Here's how the part is built. I have some questions about the finished solid (model axes, mm). A direction names the side the tool comes from. Coordinates: 2 decimals unless noted, no trailing zeros. Write each loop counter-clockwise with the first axis right and the second up, starting at its lowest first coordinate (ties: lowest second). Pieces come first, ordered by that corner, then holes. Notation, with made-up numbers: (79, 45) - (99, 45) arc R12 ccw to (99, 67) - close; hole circle Ø6 at (-34, -30.75). An arc over 180 degrees is marked (long way). Answer in a Markdown table with one row per item. Add a question column.
Item 1: I'm going to push flat-ended pins straight in: pin 1 (3 mm diameter, centred on x = 2, z = -57, fed in from +Y); pin 2 (6 mm diameter, centred on x = -2.5, y = 86, fed in from +Z); pin 3 (3 mm diameter, centred on x = 1.5, z = -199, fed in from -Y); pin 4 (3 mm diameter, centred on x = 1.5, y = 30, fed in from -Z). Where does each tip first touch, or does it pass through?
Item 2: Imagine slicing it at B-B (y = 57). Please give me the cut outline in (x, z).
Item 3: We'd pull the mould along Y, two halves only. Please class faces 3 (the face through (0.07, 7.54, -156.01)), 4 (the face through (0.07, 140.003, -241.695)), 5 (the face through (0, 20, -61)), 6 (the face through (-0.07, 81.438, -67.325)): +Y half, -Y half, draft (parallel to the pull), parting line (faces both ways), or undercut.
Item 4: Which directions (+Z, -Z, +X, -X, +Y, -Y) give clear straight access to the entire face, cutting with the end or side of a thin tool? Please do faces 1 (the face through (-0.07, 77.45, -37.26)), 2 (the face through (0.07, 144.455, -121.625)).
Item 5: Imagine slicing it at A-A (z = -275). Please give me the cut outline in (x, y).
Item 6: If I drill on probe 1 along Y at (x, z) = (-2, -70); probe 2 along Z at (x, y) = (0.5, 36); probe 3 along Z at (x, y) = (2.75, 62.5), over which ranges is the centre line in solid material (lowest first)? Write a range as from..to.
Item 7: Imagine slicing it at C-C (x = -1.25). State how many separate pieces and enclosed holes the cut face has, plus the area to 3 significant figures.
from build123d import *

# Parameters (mm, degrees)
ESQUISSE1_W                  = 300
ESQUISSE1_H                  = 150
BOSS_EXTRU_1_DEPTH           = 5
ESQUISSE2_OUTSIDE_W          = 369.112
ESQUISSE2_OUTSIDE_H          = 219.112
ENL_V_MAT_EXTRU_1_DEPTH      = 5
ENL_V_MAT_EXTRU_2_DEPTH      = 336.559234711
ENL_V_MAT_EXTRU_2_DEPTH_BACK = 336.559234711
ENL_V_MAT_EXTRU_3_DEPTH      = 336.559234711
ENL_V_MAT_EXTRU_3_DEPTH_BACK = 336.559234711
ENL_V_MAT_EXTRU_4_DEPTH      = 336.559234711
ENL_V_MAT_EXTRU_4_DEPTH_BACK = 336.559234711
ESQUISSE5_R                  = 10
ESQUISSE6_W                  = 20
ESQUISSE6_H                  = 10
ENL_V_MAT_EXTRU_5_DEPTH      = 49


with BuildPart() as part:
    # Esquisse1 → Boss.-Extru.1 (new, symmetric)
    with BuildSketch(Plane(origin=(0, 0, 0), x_dir=(0, 0, -1), z_dir=(1, 0, 0))):
        with Locations((150, 75)):
            Rectangle(ESQUISSE1_W, ESQUISSE1_H)
    extrude(amount=BOSS_EXTRU_1_DEPTH, both=True)

    # Esquisse2 outside → Enlèv. mat.-Extru.1 (cut, symmetric)
    with BuildSketch(Plane(origin=(0, 0, 0), x_dir=(0, 0, -1), z_dir=(1, 0, 0))):
        with Locations((150, 75)):
            Rectangle(ESQUISSE2_OUTSIDE_W, ESQUISSE2_OUTSIDE_H)
        Polygon((0, 117.225703003), (60, 139.063917059), (185, 150), (300, 129.722397219), (300, 99.722397219), (211.741963761, 84.160124165), (171.741963761, 14.878091862), (139.835792798, 0), (29.835792798, 0), (0, 17.225703003), align=None, mode=Mode.SUBTRACT)
    extrude(amount=ENL_V_MAT_EXTRU_1_DEPTH, both=True, mode=Mode.SUBTRACT)

    # Esquisse3 → Enlèv. mat.-Extru.2 (cut, two sides: drawn at the far end of the back side and taken through both)
    with BuildSketch(Plane(origin=(5, 0, 0), x_dir=(0, 0, -1), z_dir=(1, 0, 0)).offset(-ENL_V_MAT_EXTRU_2_DEPTH_BACK)):
        Polygon((20, 103.221552239), (20, 80.493304508), (55, 74.321860183), (80, 88.755616913), (62.679491924, 118.755616913), align=None)
        Polygon((90, 71.435108837), (113.922571241, 30), (81.508057782, 49.831775443), align=None)
        Polygon((82.886751346, 123.755616913), (139.903333355, 25), (175.32640016, 86.354551467), (150.32640016, 129.655821657), align=None)
        Polygon((91.944969354, 20), (30, 20), (30, 48.267236345), (52.117107943, 44.367393479), align=None)
    extrude(amount=ENL_V_MAT_EXTRU_2_DEPTH + ENL_V_MAT_EXTRU_2_DEPTH_BACK, mode=Mode.SUBTRACT)

    # Esquisse4 → Enlèv. mat.-Extru.3 (cut, two sides: drawn at the far end of the back side and taken through both)
    with BuildSketch(Plane(origin=(5, 0, 0), x_dir=(0, 0, -1), z_dir=(1, 0, 0)).offset(-ENL_V_MAT_EXTRU_3_DEPTH_BACK)):
        Polygon((0, 97.225703003), (3, 97.225703003), (5, 99.225703003), (5, 91.225703003), (3, 93.225703003), (0, 93.225703003), align=None)
        Polygon((3, 41.225703003), (0, 41.225703003), (0, 37.225703003), (3, 37.225703003), (5, 35.225703003), (5, 43.225703003), align=None)
    extrude(amount=ENL_V_MAT_EXTRU_3_DEPTH + ENL_V_MAT_EXTRU_3_DEPTH_BACK, mode=Mode.SUBTRACT)

    # Esquisse5 → Enlèv. mat.-Extru.4 (cut, two sides: drawn at the far end of the back side and taken through both)
    with BuildSketch(Plane.ZY.offset(5).offset(-ENL_V_MAT_EXTRU_4_DEPTH_BACK)):
        with Locations((-275, 114.722397219)):
            Circle(ESQUISSE5_R)
    extrude(amount=ENL_V_MAT_EXTRU_4_DEPTH + ENL_V_MAT_EXTRU_4_DEPTH_BACK, mode=Mode.SUBTRACT)

    # Esquisse6 → Enlèv. mat.-Extru.5 (cut)
    with BuildSketch(Plane(origin=(5, 0, 0), x_dir=(0, 0, -1), z_dir=(1, 0, 0))):
        with Locations((195, 128)):
            Rectangle(ESQUISSE6_W, ESQUISSE6_H)
    extrude(amount=-ENL_V_MAT_EXTRU_5_DEPTH, mode=Mode.SUBTRACT)


solid = part.part
Here are the results:
| question | item | result |
|---|---|---|
| 1 | pin 1 | stops at y = 138.52 |
| 1 | pin 2 | stops at z = 0 |
| 1 | pin 3 | stops at y = 59.49 |
| 1 | pin 4 | stops at z = -181.34 |
| 2 | outline | (-5, -196.06) - (5, -196.06) - (5, -158.38) - (-5, -158.38) - close; (-5, -121.43) - (5, -121.43) - (5, -98.33) - (-5, -98.33) - close; (-5, -84.33) - (5, -84.33) - (5, 0) - (-5, 0) - close |
| 3 | face 3 | -Y half |
| 3 | face 4 | +Y half |
| 3 | face 5 | undercut |
| 3 | face 6 | undercut |
| 4 | face 1 | +X, -X |
| 4 | face 2 | +Z, +X, -X, +Y |
| 5 | outline | (-5, 95.31) - (5, 95.31) - (5, 104.72) - (-5, 104.72) - close; (-5, 124.72) - (5, 124.72) - (5, 134.13) - (-5, 134.13) - close |
| 6 | probe 1 | y = 0..20, 33.43..82.98, 106.08..139.94 |
| 6 | probe 2 | z = -183.94..-146.25, -133.55..-110.46, -104.12..-65.79, -30..-5, -4.23..0 |
| 6 | probe 3 | z = -199.24..-161.55, -118.25..-95.16, -86.49..0 |
| 7 | separate pieces | 1 |
| 7 | enclosed holes | 6 |
| 7 | area | 22,400 mm2 |
